The model under review builds one solid part; all positions refer to its coordinate system, in mm. Round coordinates to 2 decimals unless told otherwise and drop trailing zeros. Write each loop counter-clockwise with the first axis right and the second up, starting at its lowest first coordinate (ties: lowest second). Pieces come first, ordered by that corner, then holes. Notation, with made-up numbers: M 18,32.5 L 40,32.5 A22 cw 40,52.5 Z; hole C 88.25,-2.5 d1. An arc over 180 degrees is marked long. One line per item, written item: value. Start each with the question number.
1) Take a section at B-B, the plane z = -26. Write out the cut boundary in (x, y), and give its area (3 significant figures).
2) Wall thickness on probe 1 along X at (y, z) = (1.6, -277); probe 2 along X at (y, z) = (3.25, -278); probe 3 along Z at (x, y) = (430, 1.65): over which ranges is each line inside the solid? List them lowest first.
3) Take a section at A-A, the plane z = -277. Write out the cut boundary in (x, y).
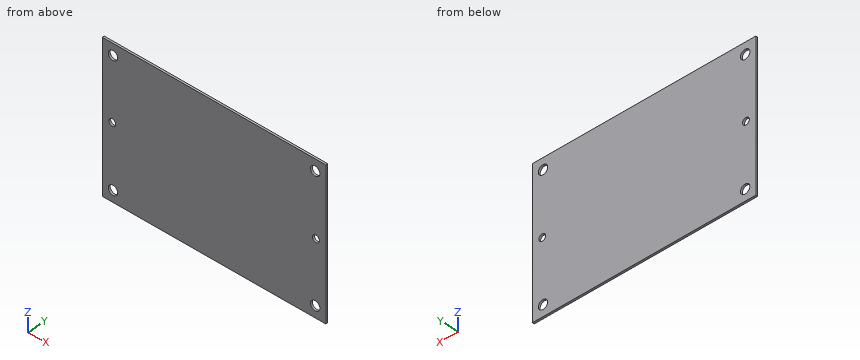
from build123d import *

# Parameters (mm, degrees)
SKETCH_1_W          = 450
SKETCH_1_H          = 300
EXTRUDE_1_DEPTH     = 4
SKETCH_2_R          = 9.5
SKETCH_2_R_2        = 7
CUT_EXTRUDE_1_DEPTH = 10


with BuildPart() as part:
    # Эскиз1 → Бобышка-Вытянуть1 (new body)
    with BuildSketch(Plane(origin=(0, 0, 0), x_dir=(1, 0, 0), z_dir=(0, 1, 0))):
        with Locations((225, 150)):
            Rectangle(SKETCH_1_W, SKETCH_1_H)
    extrude(amount=EXTRUDE_1_DEPTH)

    # Эскиз2 → Вырез-Вытянуть1 (cut)
    with BuildSketch(Plane(origin=(0, 4, 0), x_dir=(1, 0, 0), z_dir=(0, 1, 0))):
        with Locations(Location((21.5, 23, 0), (0, 0, 270))):
            Circle(SKETCH_2_R)
        with Locations(Location((20, 150, 0), (0, 0, 270))):
            Circle(SKETCH_2_R_2)
        with Locations(Location((21.5, 277, 0), (0, 0, 270))):
            Circle(SKETCH_2_R)
        with Locations(Location((428.5, 23, 0), (0, 0, 270))):
            Circle(SKETCH_2_R)
        with Locations(Location((430, 150, 0), (0, 0, 270))):
            Circle(SKETCH_2_R_2)
        with Locations(Location((428.5, 277, 0), (0, 0, 270))):
            Circle(SKETCH_2_R)
    extrude(amount=-CUT_EXTRUDE_1_DEPTH, mode=Mode.SUBTRACT)


solid = part.part
Checked values:
1. outline: M 0,0 L 12.49,0 L 12.49,4 L 0,4 Z; M 30.51,0 L 419.49,0 L 419.49,4 L 30.51,4 Z; M 437.51,0 L 450,0 L 450,4 L 437.51,4 Z
1. area: 1,660 mm2
2. probe 1: x = 0 to 12, 31 to 419, 438 to 450
2. probe 2: x = 0 to 12.05, 30.95 to 419.05, 437.95 to 450
2. probe 3: z = -300 to -286.38, -267.62 to -157, -143 to -32.38, -13.62 to 0
3. outline: M 0,0 L 12,0 L 12,4 L 0,4 Z; M 31,0 L 419,0 L 419,4 L 31,4 Z; M 438,0 L 450,0 L 450,4 L 438,4 Z
